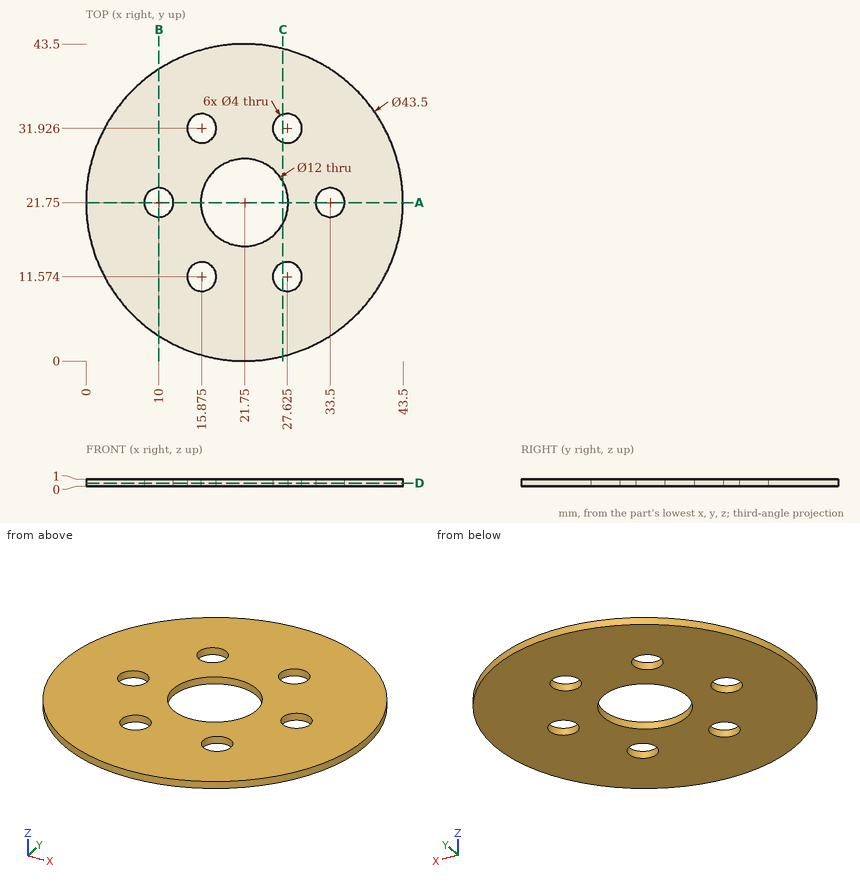
The figure shows three views and two pictorial views of one solid part (mm, origin at its lowest corner). Answer the questions. Give positions to 0.01 mm unless a question says otherwise; leave off trailing zeros. Write each loop counter-clockwise with the first axis right and the second up, starting at its lowest first coordinate (ties: lowest second). Pieces come first, ordered by that corner, then holes. Notation, with made-up numbers: (77, -5) -> (124, -5) arc R28 cw to (124, 26) -> close; hole circle Ø10 at (-17.75, 16). An arc over 180 degrees is marked (long way). Answer as a JSON object with one key per item and string values.
1) Section B-B on x = 10 is taken. Write down the section's boundary in (y, z).
Findings below:
{"outline": "(3.45, 0) -> (19.75, 0) -> (19.75, 1) -> (3.45, 1) -> close; (23.75, 0) -> (40.05, 0) -> (40.05, 1) -> (23.75, 1) -> close"}
2) Straight lines are drawn through the part: probe 1 along Y at (x, z) = (21.75, 0.55); probe 2 along X at (y, z) = (11.5, 0.2); probe 3 along Y at (x, z) = (28.5, 0.95) (1 decimal). For each, find the intervals that lie inside material, in ascending order. Write a range as from..to.
Findings below:
{"probe 1": "y = 0..15.75, 27.75..43.5", "probe 2": "x = 2.57..13.88, 17.87..25.63, 29.62..40.93", "probe 3": "y = 1.1..9.8, 13.4..30.1, 33.7..42.4"}
3) Section D-D on z = 0.45 is taken. Count the separate pieces of the cut face and the enclosed holes in it, then the cut area to 3 significant figures.
Findings below:
{"separate pieces": "1", "enclosed holes": "7", "area": "1,300 mm^2"}
4) Section C-C on x = 27 is taken. Write down the section's boundary in (y, z) (1 decimal).
Findings below:
{"outline": "(0.6, 0) -> (9.7, 0) -> (9.7, 1) -> (0.6, 1) -> close; (13.5, 0) -> (18.8, 0) -> (18.8, 1) -> (13.5, 1) -> close; (24.7, 0) -> (30, 0) -> (30, 1) -> (24.7, 1) -> close; (33.8, 0) -> (42.9, 0) -> (42.9, 1) -> (33.8, 1) -> close"}
5) Section A-A on y = 21.75 is taken. Write down the section's boundary in (x, z), then the cut area to 3 significant figures.
Findings below:
{"outline": "(0, 0) -> (8, 0) -> (8, 1) -> (0, 1) -> close; (12, 0) -> (15.75, 0) -> (15.75, 1) -> (12, 1) -> close; (27.75, 0) -> (31.5, 0) -> (31.5, 1) -> (27.75, 1) -> close; (35.5, 0) -> (43.5, 0) -> (43.5, 1) -> (35.5, 1) -> close", "area": "23.5 mm^2"}
